The model under review builds one solid part; all positions refer to its coordinate system, in mm. A direction names the side the tool comes from. Round coordinates to 2 decimals unless told otherwise and drop trailing zeros. Loops run counter-clockwise (first coordinate to the right, second up) from the corner with the lowest first, then second, coordinate; pieces in that order, holes last. Notation, with made-up numbers: (60, -38.75) -> (100, -38.75) arc R17 cw to (100, -17.75) -> close; hole circle Ø10 at (10, 24.5). An arc over 180 degrees is marked (long way). Write each question's results on one line, items separated by ' | '. Start each with the question number.
Item 1: We need section A-A (x = 37). Give the boundary of the cut face in (y, z), and give its area (3 significant figures).
Item 2: Clearance check with flat-ended pins moving along their axes: pin 1 Ø6 at (x, y) = (99.468, 11) entering from -Z; pin 2 Ø0.9 at (x, z) = (-165.5, -1) entering from +Y; pin 3 Ø2.5 at (x, z) = (-37, -5.5) entering from +Y. State where each tip first meets the part, or that it passes through.
Item 3: We need section B-B (z = -5.5). Give the boundary of the cut face in (x, y).
Item 4: Tool access review of faces 1 (the flat face through (3, 17, -3.048)), 2 (the flat face through (190.5, 5, -2)): name each direction out of +Z, -Z, +X, -X, +Y, -Y from which nothing blocks a thin tool from reaching the whole face with its end or side.
Item 5: For L1, parallel to Y at x = 135.9, z = -1.7; L2, parallel to X at y = 10, z = -1.5; L3, parallel to Z at x = 73.5, y = 28, list the stretches that pass through material, from the lowest coordinate up. Write a range as from..to.
from build123d import *

# Parameters (mm, degrees)
BOSS_EXTRUDE1_DEPTH     = 190.5
F_6_CLEARANCE_HOLE1_D   = 3.7973
CUT_EXTRUDE1_DEPTH      = 32.75
SKETCH6_W               = 25.4
SKETCH6_H               = 15.24
CUT_EXTRUDE2_DEPTH      = 191.5
CUT_EXTRUDE2_DEPTH_BACK = 191.5


with BuildPart() as part:
    # Sketch1 → Boss-Extrude1 (new body, symmetric)
    with BuildSketch(Plane(origin=(0, 0, 0), x_dir=(0, 0, -1), z_dir=(1, 0, 0))):
        Polygon((0, 0), (31.75, 0), (31.75, 3.048), (3.048, 3.048), (3.048, 31.75), (0, 31.75), align=None)
    extrude(amount=BOSS_EXTRUDE1_DEPTH, both=True)

    # #6 Clearance Hole1 (through all)
    with Locations(Plane.XY):
        with Locations((135.9, 27), (135.9, 11), (99.5, 27), (99.468, 11), (-121.868, 27), (-121.868, 11), (-85.468, 11), (-85.468, 27)):
            Hole(F_6_CLEARANCE_HOLE1_D / 2)

    # Sketch5 → Cut-Extrude1 (cut, through all)
    with BuildSketch(Plane.XY):
        with BuildLine():
            Line((149.877, 41.148), (149.877, 19.558))
            ThreePointArc((149.877, 19.558), (150.992923164, 16.863923164), (153.687, 15.748))
            Line((153.687, 15.748), (186.69, 15.748))
            ThreePointArc((186.69, 15.748), (189.384076836, 14.632076836), (190.5, 11.938))
            Line((190.5, 11.938), (190.5, -9.652))
            Line((190.5, -9.652), (198.12, -9.652))
            Line((198.12, -9.652), (198.12, 41.148))
            Line((198.12, 41.148), (149.877, 41.148))
        make_face()
        with BuildLine():
            Line((-198.12, 41.148), (-149.877, 41.148))
            Line((-149.877, 41.148), (-149.877, 19.558))
            ThreePointArc((-149.877, 19.558), (-150.992923164, 16.863923164), (-153.687, 15.748))
            Line((-153.687, 15.748), (-186.69, 15.748))
            ThreePointArc((-186.69, 15.748), (-189.384076836, 14.632076836), (-190.5, 11.938))
            Line((-190.5, 11.938), (-190.5, -9.652))
            Line((-190.5, -9.652), (-198.12, -9.652))
            Line((-198.12, -9.652), (-198.12, 41.148))
        make_face()
    extrude(amount=-CUT_EXTRUDE1_DEPTH, mode=Mode.SUBTRACT)

    # Sketch6 → Cut-Extrude2 (cut, two sides)
    with BuildSketch(Plane(origin=(0, 0, 0), x_dir=(0, 0, -1), z_dir=(1, 0, 0))) as cut_extrude2_sk:
        with Locations((20.32, 0)):
            Rectangle(SKETCH6_W, SKETCH6_H)
    extrude(amount=CUT_EXTRUDE2_DEPTH, mode=Mode.SUBTRACT)
    extrude(cut_extrude2_sk.sketch, amount=-CUT_EXTRUDE2_DEPTH_BACK, mode=Mode.SUBTRACT)


solid = part.part
Here are the results:
1) outline: (0, -7.62) -> (3.05, -7.62) -> (3.05, -3.05) -> (31.75, -3.05) -> (31.75, 0) -> (0, 0) -> close | area: 111 mm2
2) pin 1: stops at z = -3.05 | pin 2: stops at y = 15.75 | pin 3: stops at y = 3.05
3) outline: (-190.5, 0) -> (190.5, 0) -> (190.5, 3.05) -> (-190.5, 3.05) -> close
4) face 1: -Z, +X, -X, +Y | face 2: +Z, -Z, +X, +Y, -Y
5) L1: y = 0..9.1, 12.9..25.1, 28.9..31.75 | L2: x = -190.5..-123.48, -120.25..-87.08, -83.85..97.85, 101.08..134.29, 137.51..190.5 | L3: z = -3.05..0
